from build123d import *

# Parameters (mm, degrees)
PAD_DEPTH    = 7
POCKET_DEPTH = 6


with BuildPart() as part:
    # Sketch → Pad (new body)
    with BuildSketch(Plane.XY):
        with BuildLine():
            Line((-23.833245, 16), (-23.833245, -16))
            Line((-23.833245, -16), (-16.062145, -17.9))
            ThreePointArc((-16.062145, -17.9), (0.222316, -24.048972), (16.390317, -17.6))
            Line((16.390317, -17.6), (25.389067, -17.45))
            Line((25.389067, 17.45), (25.389067, -17.45))
            Line((16.390317, 17.6), (25.389067, 17.45))
            ThreePointArc((16.390317, 17.6), (0.222316, 24.048972), (-16.062145, 17.9))
            Line((-23.833245, 16), (-16.062145, 17.9))
        make_face()
    extrude(amount=PAD_DEPTH)

    # Sketch001 → Pocket (cut)
    with BuildSketch(Plane.XY):
        with BuildLine():
            Line((-16.329115, 16.9), (-25.652205, 15.7))
            Line((-25.652205, 15.7), (-25.652205, -15.7))
            Line((-25.652205, -15.7), (-16.329115, -16.9))
            ThreePointArc((-16.329115, -16.9), (-0.108455, -23.49975), (16.17243, -17.05))
            Line((16.17243, -17.05), (25.659263, -16.55))
            Line((25.659263, 16.55), (25.659263, -16.55))
            Line((16.17243, 17.05), (25.659263, 16.55))
            ThreePointArc((16.17243, 17.05), (-0.108455, 23.49975), (-16.329115, 16.9))
        make_face()
    extrude(amount=POCKET_DEPTH, mode=Mode.SUBTRACT)


solid = part.part
Design review of the part built by this model. Coordinates are the model's own, in mm. A direction names the side the tool comes from. Give positions to 0.01 mm unless a question says otherwise; leave off trailing zeros. Loops run counter-clockwise (first coordinate to the right, second up) from the corner with the lowest first, then second, coordinate; pieces in that order, holes last. Notation, with made-up numbers: (49.5, 79.25) - (91.5, 79.25) arc R34 cw to (91.5, 114.25) - close; hole circle Ø11 at (82, 85). An arc over 180 degrees is marked (long way). Use CSV: the item, a comma, the result in double quotes. Start each with the question number.
1. Add section D-D (y = -8). State the section outline as (x, z) points, plus the area to 3 significant figures.
2. Machinability: for faces 4 (the flat face through (-20.002, 16.937, 3.451)), 5 (the flat face through (-20.13, -16.41, 2.96)), which of the approach directions +Z, -Z, +X, -X, +Y, -Y give a long, thin tool a straight path to every point of the face, cutting with its end or side? Answer none if there is none.
3. Add section B-B (x = -1.5). State the section outline as (y, z) points, plus the area to 3 significant figures.
4. Add section C-C (y = -20.5). State the section outline as (x, z) points, plus the area to 3 significant figures.
5. Insertion check: P1, Ø1.5, axis at x = -17, z = 1.5, coming from the +Y side; P2, Ø4, axis at y = -1.5, z = 2.5, coming from the +X side; P3, Ø4, axis at x = 11, y = 15, coming from the -Z side. Each pin has a flat end and moves straight along its axis. Give the tip position at first contact, or say it passes through.
6. Wall thickness on L1, parallel to Y at x = -8, z = 5.5; L2, parallel to Z at x = -3, y = 19; L3, parallel to X at y = -18, z = 0.75: over which ranges is each line inside the solid? List them lowest first.
7. Add section A-A (z = 1.75). State the section outline as (x, y) points.
8. Draft analysis for pull direction X (two halves, no side actions). For faces 1 (the flat face through (-20.002, -16.937, 3.451)), 2 (the flat face through (0, 0, 7)), 3 (the cylindrical face through (0.1, 23.5, 3)), state which applies: released by +X, released by -X, zero draft, split by the parting line, or undercut.
Results found:
1,outline,"(-23.83, 6) - (25.39, 6) - (25.39, 7) - (-23.83, 7) - close"
1,area,"49.2 mm²"
2,face 4,"+Z, -Z, -X, +Y"
2,face 5,"-Z"
3,outline,"(-24, 0) - (-23.45, 0) - (-23.45, 6) - (23.45, 6) - (23.45, 0) - (24, 0) - (24, 7) - (-24, 7) - close"
3,area,"54.6 mm²"
4,outline,"(-12.58, 0) - (-11.49, 0) - (-11.49, 6) - (11.49, 6) - (11.49, 0) - (12.58, 0) - (12.58, 7) - (-12.58, 7) - close"
4,area,"38.2 mm²"
5,P1,"stops at y = 17.85"
5,P2,"passes through"
5,P3,"stops at z = 6"
6,L1,"y = -22.68 to -22.1, 22.1 to 22.68"
6,L2,"z = 6 to 7"
6,L3,"x = -15.95 to -15.11, 15.11 to 15.95"
7,outline,"(-23.83, -16) - (-16.06, -17.9) arc R24.05 ccw to (16.39, -17.6) - (25.39, -17.45) - (25.39, -16.56) - (16.17, -17.05) arc R23.5 cw to (-16.33, -16.9) - (-23.83, -15.93) - close; (-23.83, 15.93) - (-16.33, 16.9) arc R23.5 cw to (16.17, 17.05) - (25.39, 16.56) - (25.39, 17.45) - (16.39, 17.6) arc R24.05 ccw to (-16.06, 17.9) - (-23.83, 16) - close"
8,face 1,"released by -X"
8,face 2,"zero draft"
8,face 3,"undercut"
